```python
from build123d import *

# Parameters (mm, degrees)
F0_W        = 38.6806862377
F0_H        = 6.35
F1_DEPTH    = 38.1
F2_T1_DEPTH = 38.1
F2_T3_DEPTH = 56.4963073453
F3_R        = 3.175
F4_DEPTH    = 25.4


# Not quite as in the source:
# - a fillet or chamfer that OpenCascade refuses, or shapes differently, is made with other operations: its cross-section is extruded or revolved along the edge and cut away or added


with BuildPart() as f1:
    # F0 (on Top) → F1 (new body)
    with BuildSketch(Plane.XY):
        Polygon((-10.8904888918, 145.4896045446), (-17.2404888918, 145.4896045446), (-17.2404888918, -57.7103954554), (-10.8904888918, -57.7103954554), (-10.8904888918, -51.3603954554), align=None)
        with Locations((8.449854227, -54.5353954554)):
            Rectangle(F0_W, F0_H)
        Polygon((27.7901973458, -22.8552754367), (27.7901973458, -51.3603954554), (27.7901973458, -57.7103954554), (34.1401973458, -57.7103954554), (34.1401973458, -22.8552754367), align=None)
    extrude(amount=F1_DEPTH)

    # F2: fillet of radius 3.6792614691 on 8 edges, made by hand

    # F2_s2 → F2_t1 (join)
    with BuildSketch(Plane.XY):
        with BuildLine():
            ThreePointArc((-7.2112274228, -51.3603954554), (-9.8128581573, -50.2827647208), (-10.8904888918, -47.6811339863))
            Line((-10.8904888918, -47.6811339863), (-10.8904888918, -51.3603954554))
            Line((-10.8904888918, -51.3603954554), (-7.2112274228, -51.3603954554))
        make_face()
        with BuildLine():
            ThreePointArc((27.7901973458, -47.6811339863), (26.7125666113, -50.2827647208), (24.1109358768, -51.3603954554))
            Line((24.1109358768, -51.3603954554), (27.7901973458, -51.3603954554))
            Line((27.7901973458, -51.3603954554), (27.7901973458, -47.6811339863))
        make_face()
    extrude(amount=F2_T1_DEPTH)

    # F2_s4 → F2_t3 (cut)
    with BuildSketch(Plane.XY.offset(-9.1981536726)):
        with BuildLine():
            ThreePointArc((31.4694588149, -22.8552754367), (28.8678280803, -23.9329061712), (27.7901973458, -26.5345369057))
            Line((27.7901973458, -26.5345369057), (27.7901973458, -22.8552754367))
            Line((27.7901973458, -22.8552754367), (31.4694588149, -22.8552754367))
        make_face()
        with BuildLine():
            ThreePointArc((34.1401973458, -26.5345369057), (33.0625666113, -23.9329061712), (30.4609358768, -22.8552754367))
            Line((30.4609358768, -22.8552754367), (34.1401973458, -22.8552754367))
            Line((34.1401973458, -22.8552754367), (34.1401973458, -26.5345369057))
        make_face()
        with BuildLine():
            ThreePointArc((-17.2404888918, -54.0311339863), (-16.1628581573, -56.6327647208), (-13.5612274228, -57.7103954554))
            Line((-13.5612274228, -57.7103954554), (-17.2404888918, -57.7103954554))
            Line((-17.2404888918, -57.7103954554), (-17.2404888918, -54.0311339863))
        make_face()
        with BuildLine():
            ThreePointArc((30.4609358768, -57.7103954554), (33.0625666113, -56.6327647208), (34.1401973458, -54.0311339863))
            Line((34.1401973458, -54.0311339863), (34.1401973458, -57.7103954554))
            Line((34.1401973458, -57.7103954554), (30.4609358768, -57.7103954554))
        make_face()
        with BuildLine():
            ThreePointArc((-14.5697503609, 145.4896045446), (-11.9681196264, 144.4119738101), (-10.8904888918, 141.8103430756))
            Line((-10.8904888918, 141.8103430756), (-10.8904888918, 145.4896045446))
            Line((-10.8904888918, 145.4896045446), (-14.5697503609, 145.4896045446))
        make_face()
        with BuildLine():
            ThreePointArc((-13.5612274228, 145.4896045446), (-16.1628581573, 144.4119738101), (-17.2404888918, 141.8103430756))
            Line((-17.2404888918, 141.8103430756), (-17.2404888918, 145.4896045446))
            Line((-17.2404888918, 145.4896045446), (-13.5612274228, 145.4896045446))
        make_face()
    extrude(amount=F2_T3_DEPTH, mode=Mode.SUBTRACT)

    # F3 (on face) → F4 (cut)
    with BuildSketch(Plane(origin=(-17.2404888918, 0, 0), x_dir=(0, -1, 0), z_dir=(-1, 0, 0))):
        with Locations((-134.0196450753, 19.05)):
            Circle(F3_R)
        with Locations((15.2053549247, 19.05)):
            Circle(F3_R)
    extrude(amount=-F4_DEPTH, mode=Mode.SUBTRACT)


solid = f1.part
```
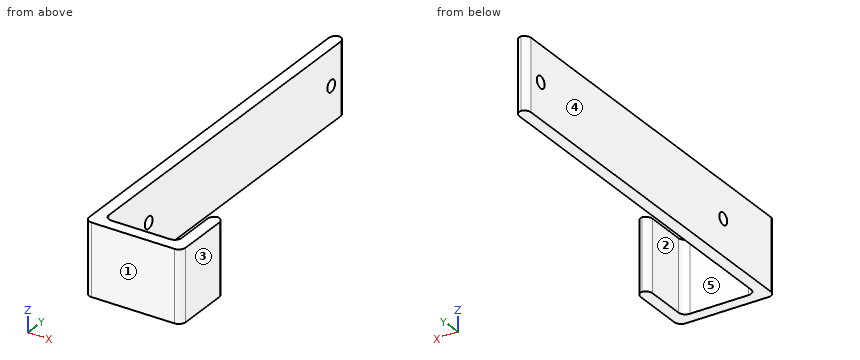
Source: CAD feature listing. Evaluate the final solid. Frame: model axes, mm. Face numbers are marked on the shaded views. A direction names the side the tool comes from. Coordinates: 2 decimals unless noted, no trailing zeros. Loops run counter-clockwise (first coordinate to the right, second up) from the corner with the lowest first, then second, coordinate; pieces in that order, holes last. Notation, with made-up numbers: M -8.5,59 L 26.5,59 A4 ccw 26.5,63 Z; hole C 39.25,71 d3. An arc over 180 degrees is marked long. Put each result on its own line as item: value. Start each with the question number.
1) Cut plane C-C on z = 11. Return the cut outline in (x, y), then the cut area to 3 significant figures.
2) Ray query, L1, parallel to Y at x = 8, z = 27.5; L2, parallel to X at y = 102, z = 15.5; L3, parallel to Y at x = -14, z = 23.5. Return the intervals inside material, ascending. Write a range as from..to.
3) Pull-direction query (X, two-part tool) for the marked faces 1, 2 and 3; classes: pulls with the +X half, pulls with the -X half, needs draft (parallel to the pull), parting line crosses it, or undercut.
4) Cut plane D-D on x = 22. Return the cut outline in (y, z), then the cut area to 3 significant figures.
5) Cut plane B-B on z = 19.05. Return the cut outline in (x, y), then the cut area to 3 significant figures.
6) Reachability of the marked faces 4 and 5 from +Z, -Z, +X, -X, +Y, -Y: full face, straight path, thin tool, end or side. Return the list, or none.
7) Contact query for flat-ended pins moving along their axis: pin 1 Ø11.5 at (y, z) = (56, 14.5) entering from +X; pin 2 Ø1 at (x, z) = (26.5, 26) entering from +Y; pin 3 Ø15.5 at (x, z) = (4.5, 20.5) entering from +Y; pin 4 Ø5.5 at (y, z) = (-15.21, 19.05) entering from +X. Output: stop coordinate, or through.
8) Cut plane A-A on y = -29.5. Return the cut outline in (x, z).
The answers:
1. outline: M -17.24,-54.03 A3.68 ccw -13.56,-57.71 L 30.46,-57.71 A3.68 ccw 34.14,-54.03 L 34.14,-26.53 A3.68 ccw 30.97,-22.89 A3.68 ccw 27.79,-26.53 L 27.79,-47.68 A3.68 cw 24.11,-51.36 L -7.21,-51.36 A3.68 cw -10.89,-47.68 L -10.89,141.81 A3.68 ccw -14.07,145.45 A3.68 ccw -17.24,141.81 Z
1. area: 1,750 mm²
2. L1: y = -57.71..-51.36
2. L2: x = -17.24..-10.89
2. L3: y = -57.68..145.45
3. face 1: needs draft
3. face 2: undercut
3. face 3: pulls with the +X half
4. outline: M -57.71,0 L -51.36,0 L -51.36,38.1 L -57.71,38.1 Z
4. area: 242 mm²
5. outline: M -17.24,-54.03 A3.68 ccw -13.56,-57.71 L 30.46,-57.71 A3.68 ccw 34.14,-54.03 L 34.14,-26.53 A3.68 ccw 30.97,-22.89 A3.68 ccw 27.79,-26.53 L 27.79,-47.68 A3.68 cw 24.11,-51.36 L -7.21,-51.36 A3.68 cw -10.89,-47.68 L -10.89,-18.38 L -17.24,-18.38 Z; M -17.24,-12.03 L -10.89,-12.03 L -10.89,130.84 L -17.24,130.84 Z; M -17.24,137.19 L -10.89,137.19 L -10.89,141.81 A3.68 ccw -14.07,145.45 A3.68 ccw -17.24,141.81 Z
5. area: 1,670 mm²
6. face 4: +Z, -Z, -X, +Y, -Y
6. face 5: +Z, -Z, +Y
7. pin 1: stops at x = -10.89
7. pin 2: stops at y = -49.96
7. pin 3: stops at y = -51.36
7. pin 4: passes through
8. outline: M -17.24,0 L -10.89,0 L -10.89,38.1 L -17.24,38.1 Z; M 27.79,0 L 34.14,0 L 34.14,38.1 L 27.79,38.1 Z
